Here's how the part is built. I have some questions about the finished solid (model axes, mm). Face numbers are marked on the shaded views. A direction names the side the tool comes from. Coordinates: 2 decimals unless noted, no trailing zeros. Loops run counter-clockwise (first coordinate to the right, second up) from the corner with the lowest first, then second, coordinate; pieces in that order, holes last. Notation, with made-up numbers: M -35,-10 L -8,-10 A19 ccw -8,13 Z; hole C 47.25,85 d4. An arc over 180 degrees is marked long. Use CSV: the item, a comma, the result in double quotes. Start each with the question number.
Q1. Which directions (+Z, -Z, +X, -X, +Y, -Y) give clear straight access to the entire face, cutting with the end or side of a thin tool? Please do the marked faces 4, 5 and 6.
Q2. For pin 1 Ø0.5 at (y, z) = (-25.5, -1) entering from +X; pin 2 Ø0.8 at (y, z) = (12.5, 9.5) entering from -X; pin 3 Ø0.5 at (y, z) = (25.5, -1.5) entering from -X, each with a flat end and sliding along its axis, tell me the tip position at first contact or that it passes through.
Q3. If we section it at D-D (y = 27): Please give me the cut outline in (x, z), and give its area (3 significant figures).
Q4. Please list where these lines run through material, in increasing order: probe 1 along X at (y, z) = (2, 3); probe 2 along Z at (x, y) = (18.5, 0.5); probe 3 along Z at (x, y) = (-15.5, 25). Write a range as [from, to].
Q5. If we section it at A-A (z = 6.5): Please give me the cut outline in (x, y).
Q6. If we section it at B-B (y = 12.5): Please give me the cut outline in (x, z).
Q7. If we mould it in two halves opening along X, with no side actions, what happens to the marked faces 1, 2 and 3? For each: +X half, -X half, draft (parallel to the pull), parting line (faces both ways), or undercut.
Q8. If we section it at C-C (x = 9): Please give me the cut outline in (y, z), and give its area (3 significant figures).
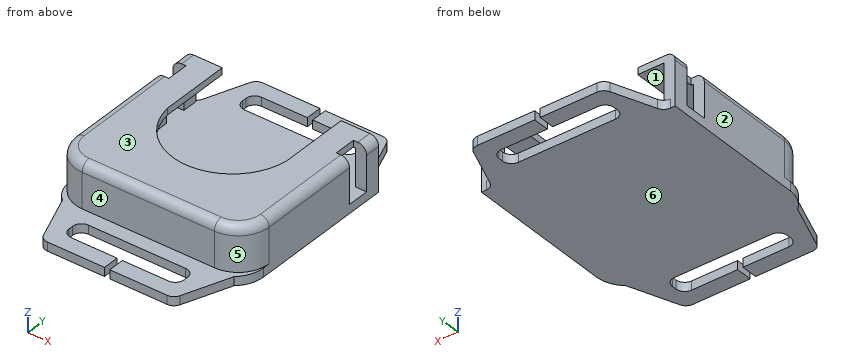
from build123d import *

# Parameters (mm, degrees)
F1_DEPTH     = 8.5
F0_W         = 39
F0_H         = 36.5
F2_DEPTH     = 1.5
F3_W         = 44
F3_H         = 39
F4_DEPTH     = 1.5
F6_DEPTH     = 2
F7_W         = 3
F7_H         = 5
F8_DEPTH     = 10
F9_R         = 7
F10_R        = 2
F0_W_2       = 26.0822549462
F0_H_2       = 5
F11_DEPTH    = 2
F12_T1_DEPTH = 28.8095132369
F13_R        = 2
F14_R        = 2
F15_W        = 1.200100407
F15_H        = 3.7374552339
F16_DEPTH    = 5


# Not quite as in the source:
# - a fillet or chamfer that OpenCascade refuses, or shapes differently, is made with other operations: its cross-section is extruded or revolved along the edge and cut away or added


with BuildPart() as f1:
    # F0 (on Top) → F1 (new body)
    with BuildSketch(Plane.XY):
        Polygon((22, -19.5), (22, 19.5), (19.5, 19.5), (19.5, -17), (-19.5, -17), (-19.5, 19.5), (-22, 19.5), (-22, -19.5), (-19.5, -19.5), (19.5, -19.5), align=None)
    extrude(amount=F1_DEPTH)

    # F0 (on Top) → F2 (join)
    with BuildSketch(Plane.XY):
        with Locations((0, 1.25)):
            Rectangle(F0_W, F0_H)
        Polygon((22, -19.5), (22, 19.5), (19.5, 19.5), (19.5, -17), (-19.5, -17), (-19.5, 19.5), (-22, 19.5), (-22, -19.5), (-19.5, -19.5), (19.5, -19.5), align=None)
    extrude(amount=-F2_DEPTH)

    # F3 (on face) → F4 (join)
    with BuildSketch(Plane.XY.offset(8.5)):
        Rectangle(F3_W, F3_H)
    extrude(amount=F4_DEPTH)

    # F5 (on face) → F6 (cut)
    with BuildSketch(Plane.XY.offset(10)):
        with BuildLine():
            Line((13.5, 3.5), (13.5, 19.5))
            Line((13.5, 19.5), (-13.5, 19.5))
            Line((-13.5, 19.5), (-13.5, 3.5))
            ThreePointArc((-13.5, 3.5), (0, -8.5), (13.5, 3.5))
        make_face()
    extrude(amount=-F6_DEPTH, mode=Mode.SUBTRACT)

    # F7 (on face) → F8 (cut)
    with BuildSketch(Plane.XY.offset(10)):
        with Locations((20.5, 13.5)):
            Rectangle(F7_W, F7_H)
        with Locations((-20.5, 13.5)):
            Rectangle(F7_W, F7_H)
    extrude(amount=-F8_DEPTH, mode=Mode.SUBTRACT)

    # F9
    f9_edges = [f1.edges().sort_by_distance(p)[0] for p in [
        (22, -19.5, 4.25),
        (-22, -19.5, 4.25),
    ]]
    fillet(f9_edges, radius=F9_R)

    # F10
    f10_edges = [f1.edges().sort_by_distance(p)[0] for p in [
        (-22, -0.75, 10),
        (-22, 17.75, 10),
        (-19.949747, -17.449747, 10),
        (0, -19.5, 10),
        (19.949747, -17.449747, 10),
        (22, -0.75, 10),
        (22, 17.75, 10),
    ]]
    fillet(f10_edges, radius=F10_R)

    # F0 (on Top) → F11 (join)
    with BuildSketch(Plane.XY):
        Polygon((22, -19.5), (22, 19.5), (19.5, 19.5), (19.5, -17), (-19.5, -17), (-19.5, 19.5), (-22, 19.5), (-22, -19.5), (-19.5, -19.5), (19.5, -19.5), align=None)
        with Locations((0, 1.25)):
            Rectangle(F0_W, F0_H)
        Polygon((-19.5, 19.5), (19.5, 19.5), (15, 31.5), (-15, 31.5), align=None)
        with Locations((0, 25.3217592835)):
            Rectangle(F0_W_2, F0_H_2, mode=Mode.SUBTRACT)
        Polygon((15, -31.5), (19.5, -19.5), (-19.5, -19.5), (-15, -31.5), align=None)
        with Locations((0, -25.3217592835)):
            Rectangle(F0_W_2, F0_H_2, mode=Mode.SUBTRACT)
    extrude(amount=-F11_DEPTH)

    # F12: fillet of radius 7 on 2 edges, made by hand

    # F12_s2 → F12_t1 (cut)
    with BuildSketch(Plane.XY.offset(-15.4047566185)):
        with BuildLine():
            ThreePointArc((-22, -14.1380973526), (-21.3442887702, -17.0961372442), (-19.5, -19.5))
            Line((-19.5, -19.5), (-19.59, -19.6072380529))
            ThreePointArc((-19.59, -19.6072380529), (-20.75, -19.64), (-22, -19.64))
            Line((-22, -19.64), (-22.14, -19.5))
            Line((-22.14, -19.5), (-22.14, -14.1380973526))
            Line((-22.14, -14.1380973526), (-22, -14.1380973526))
        make_face()
        with BuildLine():
            ThreePointArc((22, -14.1380973526), (21.3442887702, -17.0961372442), (19.5, -19.5))
            Line((19.5, -19.5), (19.59, -19.6072380529))
            ThreePointArc((19.59, -19.6072380529), (20.75, -19.64), (22, -19.64))
            Line((22, -19.64), (22.14, -19.5))
            Line((22.14, -19.5), (22.14, -14.1380973526))
            Line((22.14, -14.1380973526), (22, -14.1380973526))
        make_face()
    extrude(amount=F12_T1_DEPTH, mode=Mode.SUBTRACT)

    # F13
    f13_edges = [f1.edges().sort_by_distance(p)[0] for p in [
        (15, 31.5, -1),
        (19.5, 19.5, -1),
        (-19.5, 19.5, -1),
        (-15, 31.5, -1),
        (15, -31.5, -1),
        (-15, -31.5, -1),
    ]]
    fillet(f13_edges, radius=F13_R)

    # F14
    f14_edges = [f1.edges().sort_by_distance(p)[0] for p in [
        (-13.041127, 22.821759, -1),
        (-13.041127, 27.821759, -1),
        (13.041127, 27.821759, -1),
        (13.041127, 22.821759, -1),
        (13.041127, -27.821759, -1),
        (13.041127, -22.821759, -1),
        (-13.041127, -22.821759, -1),
        (-13.041127, -27.821759, -1),
    ]]
    fillet(f14_edges, radius=F14_R)

    # F15 (on face) → F16 (cut)
    with BuildSketch(Plane.XY):
        with Locations((-0.0326880836, 29.6578230336)):
            Rectangle(F15_W, F15_H)
        with Locations((-0.0326880836, -29.6578230336)):
            Rectangle(F15_W, F15_H)
    extrude(amount=-F16_DEPTH, mode=Mode.SUBTRACT)


solid = f1.part
Results below:
1,face 4,"+Z, +X, -X, -Y"
1,face 5,"+Z, +X, -Y"
1,face 6,"-Z, +X, -X, +Y, -Y"
2,pin 1,"x = 17.34"
2,pin 2,"x = -19"
2,pin 3,"x = -17.34"
3,outline,"M -16.69,-2 L -12.66,-2 L -12.66,0 L -16.69,0 Z; M 12.66,-2 L 16.69,-2 L 16.69,0 L 12.66,0 Z"
3,area,"16.1 mm^2"
4,probe 1,"[-22, -19.5], [19.5, 22]"
4,probe 2,"[-2, 0], [8.5, 10]"
4,probe 3,"[-2, 0]"
5,outline,"M -22,-12.5 A7 ccw -15,-19.5 L 15,-19.5 A7 ccw 22,-12.5 L 22,11 L 19.5,11 L 19.5,-17 L -19.5,-17 L -19.5,11 L -22,11 Z; M -22,16 L -19.5,16 L -19.5,19.5 L -22,19.5 Z; M 19.5,16 L 22,16 L 22,19.5 L 19.5,19.5 Z"
6,outline,"M -22,-2 L 22,-2 L 22,0 L -22,0 Z; M -19,8.5 L -13.5,8.5 L -13.5,10 L -19,10 Z; M 13.5,8.5 L 19,8.5 L 19,10 L 13.5,10 Z"
7,face 1,"undercut"
7,face 2,"-X half"
7,face 3,"draft"
8,outline,"M -31.5,-2 L -27.82,-2 L -27.82,0 L -31.5,0 Z; M -22.82,-2 L 22.82,-2 L 22.82,0 L -17,0 L -17,8.5 L -5.09,8.5 L -5.09,10 L -17.5,10 A2 ccw -19.5,8 L -19.5,0 L -22.82,0 Z; M 27.82,-2 L 31.5,-2 L 31.5,0 L 27.82,0 Z"
8,area,"148 mm^2"
